Autodesk Inventor part; units mm, degrees
ref_plane "YZ Plane" through (0, 0, 0) normal (1, 0, 0) x (0, 1, 0)
ref_plane "XZ Plane" through (0, 0, 0) normal (0, 1, 0) x (-1, 0, 0)
ref_plane "XY Plane" through (0, 0, 0) normal (0, 0, 1) x (1, 0, 0)
sketch "Sketch1" plane through (0, 0, 0) normal (0, 0, 1) x (1, 0, 0)
  line L0 (-31, -28.5) -> (31, -28.5)
  line L1 (31, -28.5) -> (31, 28.5)
  line L2 (31, 28.5) -> (-31, 28.5)
  line L3 (-31, 28.5) -> (-31, -28.5)
  line L4 (-31, -28.5) -> (31, 28.5) construction
  line L5 (31, -28.5) -> (-31, 28.5) construction
  point P0 (0, 0)
  dimension "d0" = 62
  dimension "d1" = 57
extrude "Extrusion1" add sketch "Sketch1" along normal blind 1.6
fillet "Fillet1" radius 4 4 edges at (31, 28.5, 0.8) (-31, 28.5, 0.8) (-31, -28.5, 0.8) (31, -28.5, 0.8)
sketch "Sketch2" plane through (0, 0, 1.6) normal (0, 0, 1) x (1, 0, 0)
  circle A0 centre (-27, 24.5) radius 1.6
  line L0 (-43.4, 0) -> (43.4, 0)
  line L1 (0, -39.9) -> (0, 39.9) construction
  line L2 (-31, 24.5) -> (-31, -24.5) construction
  line L3 (27, 28.5) -> (-27, 28.5) construction
  circle A1 centre (27, 24.5) radius 1.6
  circle A2 centre (-27, -24.5) radius 1.6
  line L4 (27, -28.5) -> (-27, -28.5) construction
  circle A3 centre (27, -24.5) radius 1.6
  point P0 (0, 0)
  dimension "d5" = 4
  dimension "d6" = 4
  dimension "d7" = 3.2
extrude "Extrusion2" cut sketch "Sketch2" against normal through all
sketch "Sketch3" plane through (0, 0, 1.6) normal (0, 0, 1) x (1, 0, 0)
  circle A0 centre (-27, -24.5) radius 1.6
  circle A1 centre (27, 24.5) radius 1.6
  circle A2 centre (27, -24.5) radius 1.6
  circle A3 centre (-27, 24.5) radius 1.6
  arc A4 (27, -28.5) -> (31, -24.5) centre (27, -24.5) ccw
  line L0 (31, -24.5) -> (31, 24.5)
  arc A5 (31, 24.5) -> (27, 28.5) centre (27, 24.5) ccw
  line L1 (27, 28.5) -> (-27, 28.5)
  arc A6 (-27, 28.5) -> (-31, 24.5) centre (-27, 24.5) ccw
  line L2 (-31, 24.5) -> (-31, -24.5)
  arc A7 (-31, -24.5) -> (-27, -28.5) centre (-27, -24.5) ccw
  line L3 (-27, -28.5) -> (27, -28.5)
  point P0 (0, 0)
equation "\"d6\" = d5"
properties part number "Controller_PCB"
Input: part model. Units: mm. Frame: model coordinates. Round coordinates to 2 decimals unless told otherwise and drop trailing zeros.
1) Pin query (flat end, axial travel): pin 1 (3 mm diameter, centred on x = -27, y = -24.5, fed in from -Z). Return the tip coordinate at first contact, or that it passes through.
Ans:
pin 1: passes through
2) Pull-direction query (Y, two-part tool) for faces 1 (the flat face through (0, -28.5, 1)), 2 (the flat face through (31, 0, 1)), 3 (the cylindrical face through (-28.18, 25.58, 0.81)), 4 (the cylindrical face through (-29.797, 27.359, 0.811)); classes: released by +Y, released by -Y, zero draft, split by the parting line, or undercut.
Ans:
face 1: released by -Y
face 2: zero draft
face 3: undercut
face 4: released by +Y
3) Material intervals for line 1 (Y direction, x = -27, z = 0.9); line 2 (Y direction, x = 27.5, z = 0.65), sorted ascending.
Ans:
line 1: y = -28.5 to -26.1, -22.9 to 22.9, 26.1 to 28.5
line 2: y = -28.47 to -26.02, -22.98 to 22.98, 26.02 to 28.47
